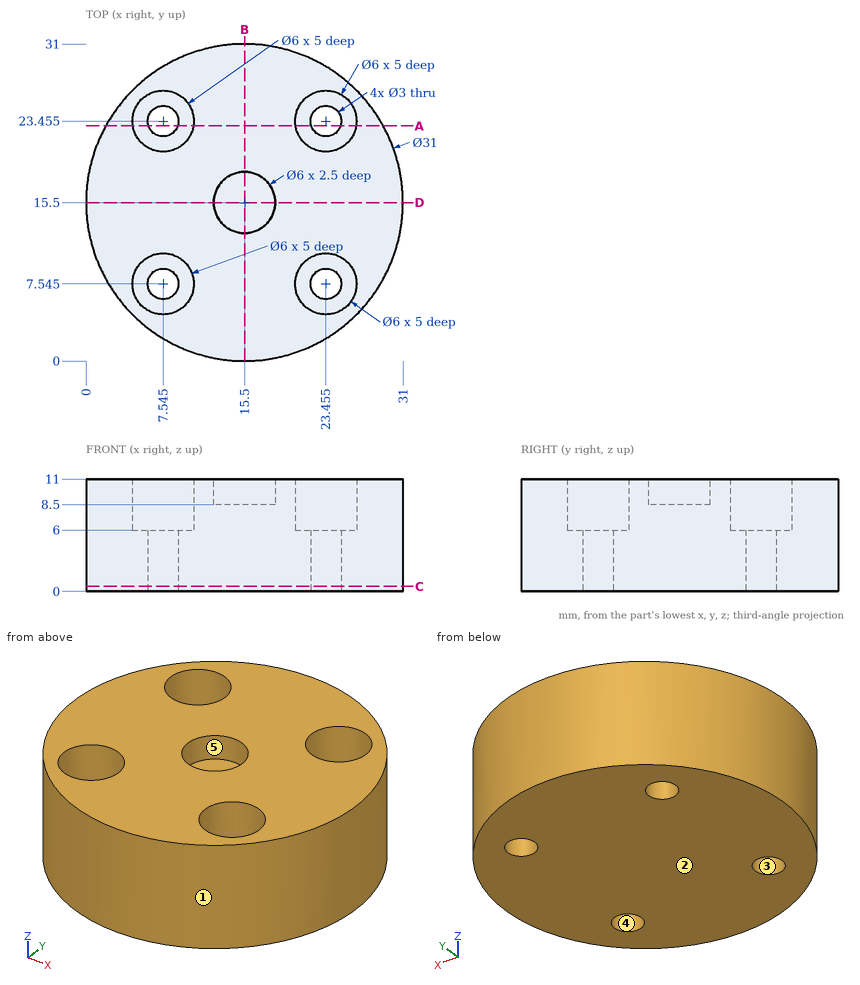
The drawing under review shows one solid part. Ordinate dimensions are in mm from its lowest x, y, z. A direction names the side the tool comes from. Round coordinates to 2 decimals unless told otherwise and drop trailing zeros. Loops run counter-clockwise (first coordinate to the right, second up) from the corner with the lowest first, then second, coordinate; pieces in that order, holes last. Notation, with made-up numbers: (-6, -37) - (53, -37) arc R20 ccw to (53, -21) - close; hole circle Ø11 at (-22, 88). An arc over 180 degrees is marked (long way). Put each result on its own line as item: value. Start each with the question number.
1. For the marked faces 4 and 5, list the 3-axis set-ups (+Z, -Z, +X, -X, +Y, -Y) from which the entire face can be reached by the end or side of a thin tool; tool diameter is ignored.
2. For probe 1 along Y at (x, z) = (21.5, 10); probe 2 along Y at (x, z) = (7, 1.25); probe 3 along Y at (x, z) = (15.5, 9.8), list the stretches that pass through material, from the lowest coordinate up. Write a range as [from, to].
3. Insertion check: P1, Ø3.5, axis at x = 23.455, y = 23.455, coming from the +Z side; P2, Ø3, axis at x = 12, z = 8, coming from the +Y side; P3, Ø2, axis at x = 13.5, z = 7.5, coming from the +Y side. Each pin has a flat end and moves straight along its axis. Give the tip position at first contact, or say it passes through.
4. Mouldability with a two-part tool opening along X and no side actions: class the marked faces 1, 2 and 3 as +X half, -X half, draft (parallel to the pull), parting line (faces both ways), or undercut.
5. Consider section B-B on x = 15.5. State the section outline as (y, z) points, plus the area to 3 significant figures.
6. Consider section A-A on y = 23. State the section outline as (x, z) points.
7. Consider section C-C on z = 0.5. State the section outline as (x, y) points (3 decimals), plus the area to 3 significant figures.
Result sheet:
1. face 4: +Z, -Z
1. face 5: +Z
2. probe 1: [1.21, 5.27], [9.82, 21.18], [25.73, 29.79]
2. probe 2: [2.54, 6.15], [8.94, 22.06], [24.85, 28.46]
2. probe 3: [0, 12.5], [18.5, 31]
3. P1: z = 6
3. P2: y = 30.87
3. P3: y = 30.97
4. face 1: parting line
4. face 2: draft
4. face 3: undercut
5. outline: (0, 0) - (31, 0) - (31, 11) - (18.5, 11) - (18.5, 8.5) - (12.5, 8.5) - (12.5, 11) - (0, 11) - close
5. area: 326 mm^2
6. outline: (1.94, 0) - (6.12, 0) - (6.12, 6) - (4.58, 6) - (4.58, 11) - (1.94, 11) - close; (8.97, 0) - (22.03, 0) - (22.03, 6) - (20.49, 6) - (20.49, 11) - (10.51, 11) - (10.51, 6) - (8.97, 6) - close; (24.88, 0) - (29.06, 0) - (29.06, 11) - (26.42, 11) - (26.42, 6) - (24.88, 6) - close
7. outline: circle Ø31 at (15.5, 15.5); hole circle Ø3 at (7.545, 7.545); hole circle Ø3 at (7.545, 23.455); hole circle Ø3 at (23.455, 7.545); hole circle Ø3 at (23.455, 23.455)
7. area: 726 mm^2
